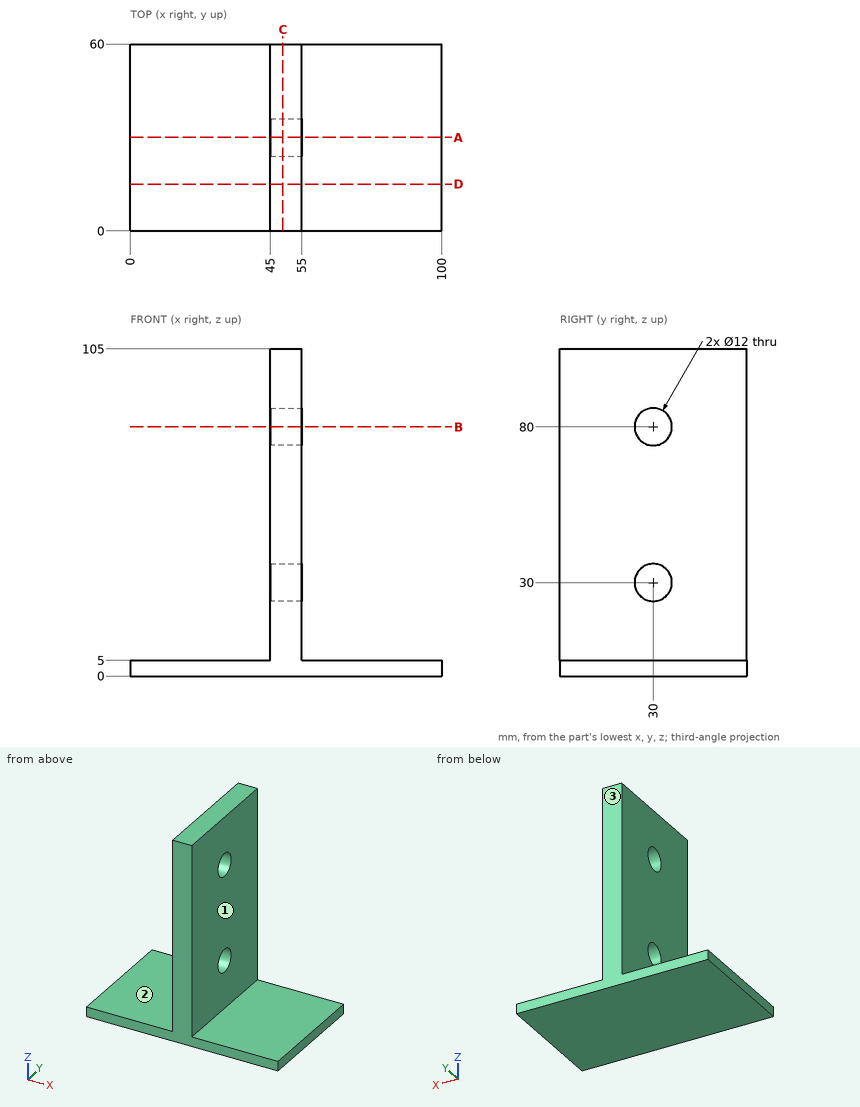
Check sheet for the drawn part. Datum: minimum x, y, z corner. Units: mm. A direction names the side the tool comes from. Coordinates: 2 decimals unless noted, no trailing zeros. Write each loop counter-clockwise with the first axis right and the second up, starting at its lowest first coordinate (ties: lowest second). Pieces come first, ordered by that corner, then holes. Notation, with made-up numbers: M 68.25,44 L 118.25,44 A7 cw 118.25,50 Z; hole C 0,80.25 d3. An arc over 180 degrees is marked long. One line per item, written item: value.
Item 1: Gauge pin test, flat ends, axial feed: pin 1 Ø22.5 at (x, y) = (12, 41.5) entering from +Z; pin 2 Ø1 at (y, z) = (15.5, 13) entering from -X; pin 3 Ø6 at (y, z) = (40.5, 83) entering from +X; pin 4 Ø11 at (y, z) = (30, 30) entering from -X. Record the tip position at first contact, or that the pin passes through.
Check sheet entries:
pin 1: stops at z = 5
pin 2: stops at x = 45
pin 3: stops at x = 55
pin 4: passes through
Item 2: Section check D-D, the plane y = 15. Record the boundary of the cut face in (x, z).
Check sheet entries:
outline: M 0,0 L 100,0 L 100,5 L 55,5 L 55,105 L 45,105 L 45,5 L 0,5 Z
Item 3: Scan lines: line 1 along Y through (x, z) = (48, 30); line 2 along Z through (x, y) = (24, 53); line 3 along X through (y, z) = (3, 87). Record each from-to range of solid material in increasing order.
Check sheet entries:
line 1: y = 0 to 24, 36 to 60
line 2: z = 0 to 5
line 3: x = 45 to 55
Item 4: Access from +Z, -Z, +X, -X, +Y, -Y to the whole of each face (thin tool, end or side, straight path). Record for the marked faces 1, 2 and 3.
Check sheet entries:
face 1: +Z, +X, +Y, -Y
face 2: +Z, -X, +Y, -Y
face 3: +Z, -Z, +X, -X, +Y
Item 5: Section check B-B, the plane z = 80. Record the boundary of the cut face in (x, y).
Check sheet entries:
outline: M 45,0 L 55,0 L 55,24 L 45,24 Z; M 45,36 L 55,36 L 55,60 L 45,60 Z
Item 6: Section check C-C, the plane x = 49. Record the boundary of the cut face in (y, z).
Check sheet entries:
outline: M 0,0 L 60,0 L 60,105 L 0,105 Z; hole C 30,30 d12; hole C 30,80 d12
Item 7: Section check A-A, the plane y = 30. Record the boundary of the cut face in (x, z), plus the area to 3 significant figures.
Check sheet entries:
outline: M 0,0 L 100,0 L 100,5 L 55,5 L 55,24 L 45,24 L 45,5 L 0,5 Z; M 45,36 L 55,36 L 55,74 L 45,74 Z; M 45,86 L 55,86 L 55,105 L 45,105 Z
area: 1,260 mm^2
